Study the drawing (mm; zero at the part's minimum x, y, z) and answer. A direction names the side the tool comes from. Coordinates: 2 decimals unless noted, no trailing zeros. Loops run counter-clockwise (first coordinate to the right, second up) from the corner with the lowest first, then second, coordinate; pieces in that order, holes last. Notation, with made-up numbers: (23, 6.5) - (55, 6.5) arc R25 ccw to (55, 32.5) - close; hole circle Ø2 at (63, 86). An arc over 180 degrees is marked (long way). Use one line per item in the form item = value.
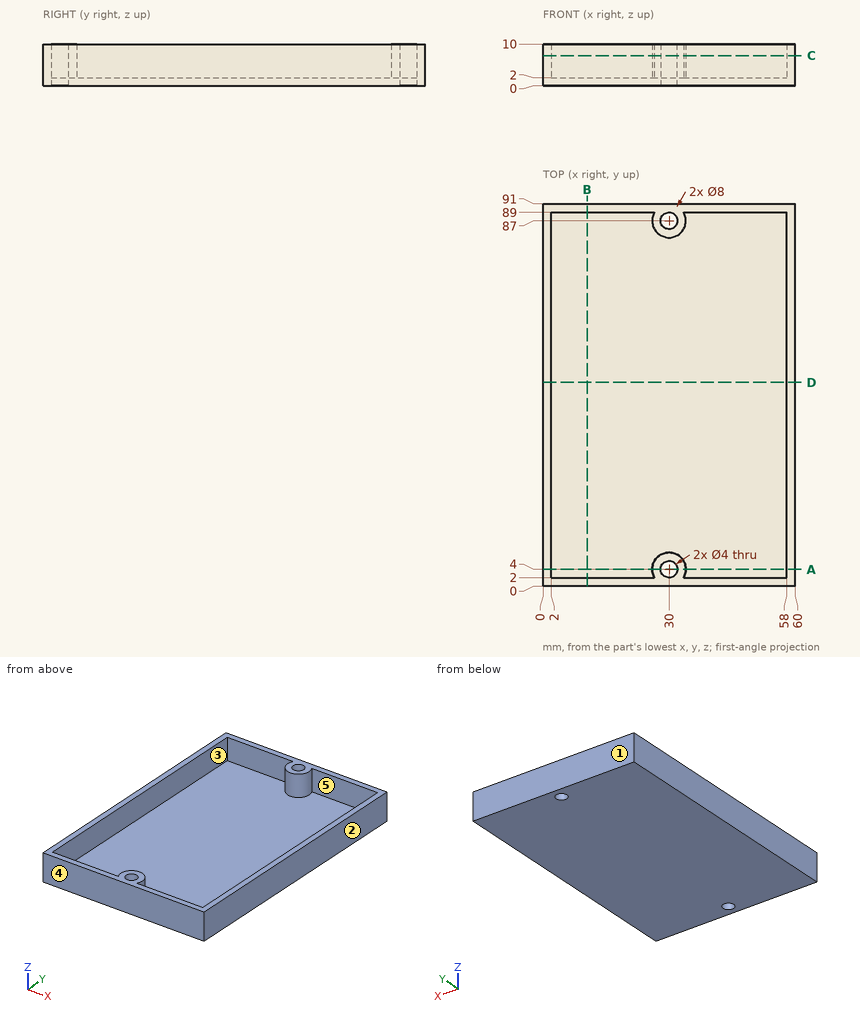
Item 1: Which of the six approach directions +Z, -Z, +X, -X, +Y, -Y give full straight-line access (tool end or side, diameter ignored) to the marked faces 4 and 5?
Results below:
face_4 = +Z, -Z, +X, -X, -Y
face_5 = +Z
Item 2: The part is cut by section A-A on y = 4. Give the vertices of the cut face in (x, z).
Results below:
outline = (0, 0) - (28, 0) - (28, 10) - (26, 10) - (26, 2) - (2, 2) - (2, 10) - (0, 10) - close; (32, 0) - (60, 0) - (60, 10) - (58, 10) - (58, 2) - (34, 2) - (34, 10) - (32, 10) - close
Item 3: For a pull along Y with two mould halves and no side action, classify the marked faces 1, 2 and 3 as +Y half, -Y half, draft (parallel to the pull), parting line (faces both ways), or undercut.
Results below:
face_1 = +Y half
face_2 = draft
face_3 = undercut
Item 4: The part is cut by section B-B on x = 10.5. Give the vertices of the cut face in (y, z), plus the area to 3 significant figures.
Results below:
outline = (0, 0) - (91, 0) - (91, 10) - (89, 10) - (89, 2) - (2, 2) - (2, 10) - (0, 10) - close
area = 214 mm²
Item 5: The part is cut by section C-C on z = 7.25. Give the vertices of the cut face in (x, y), plus the area to 3 significant figures.
Results below:
outline = (0, 0) - (60, 0) - (60, 91) - (0, 91) - close; hole (2, 2) - (26.54, 2) arc R4 cw (long way) to (33.46, 2) - (58, 2) - (58, 89) - (33.46, 89) arc R4 cw (long way) to (26.54, 89) - (2, 89) - close; hole circle Ø4 at (30, 4); hole circle Ø4 at (30, 87)
area = 644 mm²
Item 6: Each of these flat-tipped pins is pushed along its axis until it touches: P1, Ø6, axis at x = 12.5, y = 80, coming from the +Z side; P2, Ø2.5, axis at x = 11, z = 7, coming from the -Y side; P3, Ø2.5, axis at x = 30, y = 4, coming from the -Z side. Where does it stop, or does it pass through?
Results below:
P1 = 2
P2 = 0
P3 = through
Item 7: Find the intervals of material crossed by L1, parallel to X at y = 87, z = 4.25; L2, parallel to Y at x = 30, z = 7; L3, parallel to Y at x = 37.5, z = 9.5, in increasing order.
Results below:
L1 = 0 to 2, 26 to 28, 32 to 34, 58 to 60
L2 = 0 to 2, 6 to 8, 83 to 85, 89 to 91
L3 = 0 to 2, 89 to 91
Item 8: The part is cut by section D-D on y = 48.5. Give the vertices of the cut face in (x, z).
Results below:
outline = (0, 0) - (60, 0) - (60, 10) - (58, 10) - (58, 2) - (2, 2) - (2, 10) - (0, 10) - close
